from build123d import *

# Parameters (mm, degrees)
EXTRUDE_1_DEPTH     = 5
EXTRUDE_START       = 3
EXTRUDE_2_DEPTH     = 3
SKETCH_3_R          = 1.5
CUT_EXTRUDE_1_DEPTH = 30.786742017
CHAMFER_1_SIZE      = 3


with BuildPart() as part:
    # ｽｹｯﾁ1 → ﾎﾞｽ - 押し出し1 (new body)
    with BuildSketch(Plane.XY):
        with BuildLine():
            ThreePointArc((-8.5, 0), (0, 8.5), (8.5, 0))
            Line((8.5, 0), (8.5, -12))
            Line((8.5, -12), (14.5, -12))
            Line((14.5, -12), (14.5, 12))
            Line((14.5, 12), (-14.5, 12))
            Line((-14.5, 12), (-14.5, -12))
            Line((-14.5, -12), (-8.5, -12))
            Line((-8.5, -12), (-8.5, 0))
        make_face()
    extrude(amount=EXTRUDE_1_DEPTH)

    # ｽｹｯﾁ2 → ﾎﾞｽ - 押し出し2 (add)
    with BuildSketch(Plane(origin=(0, 0, 0), x_dir=(-1, 0, 0), z_dir=(0, 0, -1)).offset(EXTRUDE_START)):
        with BuildLine():
            Line((8.5, -12), (8.5, -19))
            Line((8.5, -19), (21.5, -19))
            Line((21.5, -19), (21.5, 19))
            Line((21.5, 19), (-21.5, 19))
            Line((-21.5, 19), (-21.5, -19))
            Line((-21.5, -19), (-8.5, -19))
            Line((-8.5, -19), (-8.5, -12))
            Line((-8.5, -12), (-8.5, 0))
            ThreePointArc((-8.5, 0), (0, 8.5), (8.5, 0))
            Line((8.5, 0), (8.5, -12))
        make_face()
    extrude(amount=-EXTRUDE_2_DEPTH)

    # ｽｹｯﾁ3 → ｶｯﾄ - 押し出し1 (cut, through all)
    with BuildSketch(Plane.XY.offset(5)):
        with Locations((11.5, 0)):
            Circle(SKETCH_3_R)
        with Locations((-11.5, 0)):
            Circle(SKETCH_3_R)
    extrude(amount=-CUT_EXTRUDE_1_DEPTH, mode=Mode.SUBTRACT)

    # 面取り1
    chamfer_1_edges = [part.edges().sort_by_distance(p)[0] for p in [
        (15, -19, -3),
        (21.5, 0, -3),
        (0, 19, -3),
        (-21.5, 0, -3),
        (-15, -19, -3),
    ]]
    chamfer(chamfer_1_edges, length=CHAMFER_1_SIZE - 0.0001)  # a hair under: the kernel refuses the full size


solid = part.part
The model under review builds one solid part; all positions refer to its coordinate system, in mm. A direction names the side the tool comes from. Give positions to 0.01 mm unless a question says otherwise; leave off trailing zeros. Order: outer loops, then holes, each group sorted by start corner. A loop starts at its lowest first (then second) coordinate and runs counter-clockwise, first axis right, second up. Notation, with made-up numbers: M 58.25,-28 L 97.25,-28 A20 ccw 97.25,-14 Z; hole C 19,53.5 d8. An arc over 180 degrees is marked long. Answer in a Markdown table with one row per item. Add a question column.
1. Add section D-D on z = 4.25. State the section outline as (x, y) points.
2. To check wall thickness, follow line 1 along Y through (x, z) = (-11.5, -0.5); line 2 along Z through (x, y) = (13.5, -15); line 3 along X through (y, z) = (7, 4). State the ranges of each line that lie inside material, in increasing order.
3. For pin 1 Ø3 at (y, z) = (0, -0.5) entering from -X; pin 2 Ø1.5 at (y, z) = (4, 2) entering from +X; pin 3 Ø1.5 at (x, z) = (0.5, 3.5) entering from +Y, all flat-tipped, find the tip position at first contact; note any pin that passes through.
4. Machinability: for faces 1 (the flat face through (0, 12, 2)), 2 (the flat face through (14.5, 0, 2)), 3 (the flat face through (11, -12, 2)), 4 (the flat face through (-8.5, -7, 1)), which of the approach directions +Z, -Z, +X, -X, +Y, -Y give a long, thin tool a straight path to every point of the face, cutting with its end or side? Answer none if there is none.
5. Mouldability with a two-part tool opening along X and no side actions: class faces 5 (the flat face through (20, 0.3, -1.5)), 6 (the flat face through (8.5, -8, 1)), 7 (the flat face through (0, 13, 0)) as released by +X, released by -X, zero draft, split by the parting line, or undercut.
The answers:
| question | item | result |
|---|---|---|
| 1 | outline | M -14.5,-12 L -8.5,-12 L -8.5,0 A8.5 cw 8.5,0 L 8.5,-12 L 14.5,-12 L 14.5,12 L -14.5,12 Z; hole C -11.5,0 d3; hole C 11.5,0 d3 |
| 2 | line 1 | -18.5 to -1.5, 1.5 to 18.5 |
| 2 | line 2 | -3 to 0 |
| 2 | line 3 | -14.5 to -4.82, 4.82 to 14.5 |
| 3 | pin 1 | x = -21.5 |
| 3 | pin 2 | x = 14.5 |
| 3 | pin 3 | y = 12 |
| 4 | face 1 | +Z, +X, -X, +Y |
| 4 | face 2 | +Z, +X, +Y, -Y |
| 4 | face 3 | +Z, +X, -X, -Y |
| 4 | face 4 | +Z, -Z, -Y |
| 5 | face 5 | released by +X |
| 5 | face 6 | undercut |
| 5 | face 7 | zero draft |
